Geometry: see drawing. Coordinates: mm, zero at the bounding-box minimum. A direction names the side the tool comes from. Round coordinates to 2 decimals unless told otherwise and drop trailing zeros. Write each loop counter-clockwise with the first axis right and the second up, starting at its lowest first coordinate (ties: lowest second). Pieces come first, ordered by that corner, then holes. Notation, with made-up numbers: (19.25, -21.5) -> (28.25, -21.5) arc R36 ccw to (28.25, 17.5) -> close; hole circle Ø4 at (46.25, 5.5). An arc over 180 degrees is marked (long way). Write item = value, one per line.
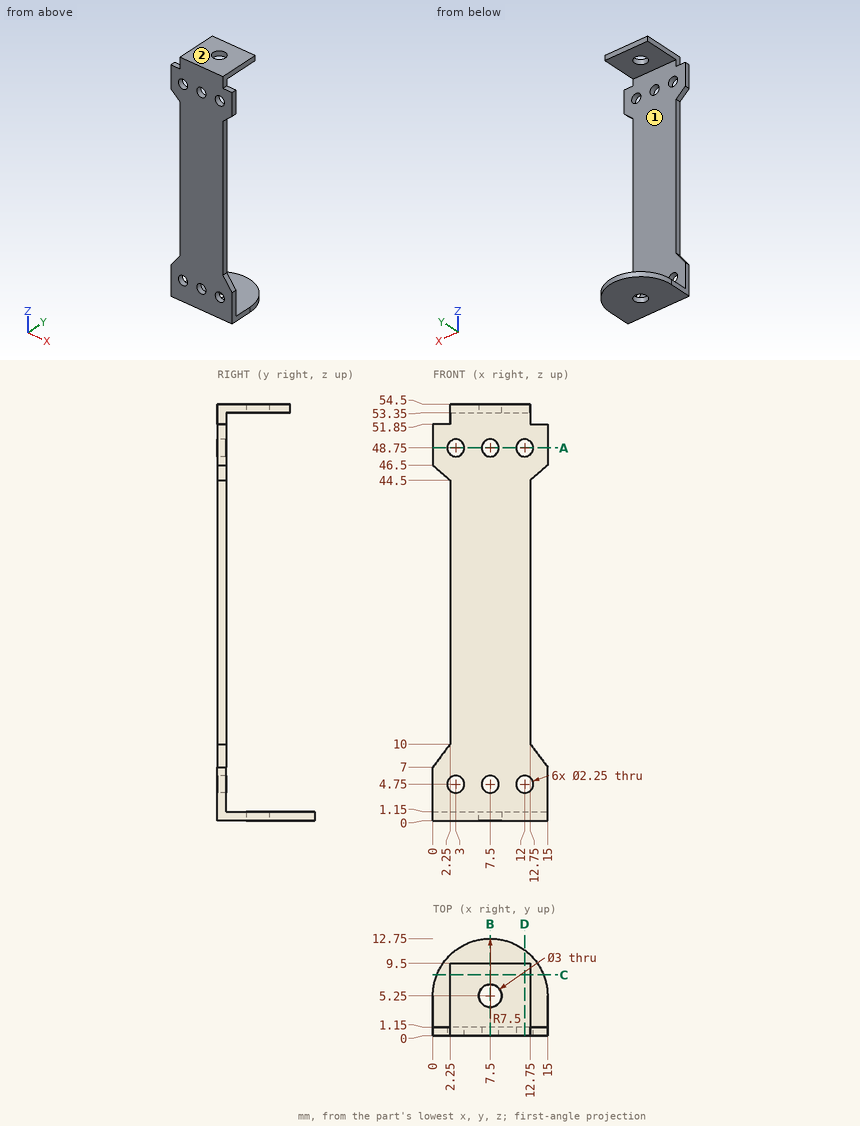
1) Line query: L1, parallel to Z at x = 7.5, y = 0.55 (3 decimals); L2, parallel to Z at x = 9.75, y = 8.75; L3, parallel to Y at x = 12, z = 22. Output: solid intervals per line, ascending. Write a range as from..to.
Solutions:
L1 = 0..3.625, 5.875..47.625, 49.875..54.5
L2 = 0..1.15, 53.35..54.5
L3 = 0..1.15
2) Cut plane D-D (x = 12). Return the cut outline in (y, z) (3 decimals).
Solutions:
outline = (0, 0) -> (11.25, 0) -> (11.25, 1.15) -> (1.15, 1.15) -> (1.15, 3.625) -> (0, 3.625) -> close; (0, 5.875) -> (1.15, 5.875) -> (1.15, 47.625) -> (0, 47.625) -> close; (0, 49.875) -> (1.15, 49.875) -> (1.15, 53.35) -> (9.5, 53.35) -> (9.5, 54.5) -> (0, 54.5) -> close
3) Access query for the marked faces 1 and 2. Directions: +Z, -Z, +X, -X, +Y, -Y. A direction counts if a zero-diameter tool reaches every point of the face in a straight line with its end or side. Return the directions, or none.
Solutions:
face_1 = +X, -X, +Y
face_2 = +Z, +X, -X, +Y, -Y
4) Cut plane A-A (z = 48.75). Return the cut outline in (x, y) (3 decimals), and give its area (3 significant figures).
Solutions:
outline = (0, 0) -> (1.875, 0) -> (1.875, 1.15) -> (0, 1.15) -> close; (4.125, 0) -> (6.375, 0) -> (6.375, 1.15) -> (4.125, 1.15) -> close; (8.625, 0) -> (10.875, 0) -> (10.875, 1.15) -> (8.625, 1.15) -> close; (13.125, 0) -> (15, 0) -> (15, 1.15) -> (13.125, 1.15) -> close
area = 9.49 mm^2
5) Cut plane B-B (x = 7.5). Return the cut outline in (y, z) (3 decimals).
Solutions:
outline = (0, 0) -> (3.75, 0) -> (3.75, 1.15) -> (1.15, 1.15) -> (1.15, 3.625) -> (0, 3.625) -> close; (0, 5.875) -> (1.15, 5.875) -> (1.15, 47.625) -> (0, 47.625) -> close; (0, 49.875) -> (1.15, 49.875) -> (1.15, 53.35) -> (3.75, 53.35) -> (3.75, 54.5) -> (0, 54.5) -> close; (6.75, 0) -> (12.75, 0) -> (12.75, 1.15) -> (6.75, 1.15) -> close; (6.75, 53.35) -> (9.5, 53.35) -> (9.5, 54.5) -> (6.75, 54.5) -> close
6) First-contact query: P1, Ø7.5, axis at x = 10.5, z = 36, coming from the +Y side; P2, Ø2, axis at y = 7, z = 54, coming from the +X side; P3, Ø1.3, axis at x = 1.5, y = 1, coming from the +Z side. Flat tips, straight axial feed; report the tip coordinate or a pass-through.
Solutions:
P1 = 1.15
P2 = 12.75
P3 = 51.85
7) Cut plane C-C (y = 8). Return the cut outline in (x, z).
Solutions:
outline = (0.52, 0) -> (14.48, 0) -> (14.48, 1.15) -> (0.52, 1.15) -> close; (2.25, 53.35) -> (12.75, 53.35) -> (12.75, 54.5) -> (2.25, 54.5) -> close
